CAD build for the part. Positions are in the model's coordinates, mm. A direction names the side the tool comes from. Round coordinates to 2 decimals unless told otherwise and drop trailing zeros. Order: outer loops, then holes, each group sorted by start corner. A loop starts at its lowest first (then second) coordinate and runs counter-clockwise, first axis right, second up. Notation, with made-up numbers: (-13.75, 85) - (27.25, 85) arc R25 ccw to (27.25, 114) - close; hole circle Ø3 at (85.25, 73.25). An arc over 180 degrees is marked (long way). Use one line per item in the form item = value. Start each with the question number.
from build123d import *

# Parameters (mm, degrees)
SKETCH_1_W               = 20
SKETCH_1_H               = 10
EXTRUDE_1_DEPTH          = 90
EXTRUDE_START            = -5
SKETCH_2_W               = 10
SKETCH_2_H               = 10
SKETCH_2_W_2             = 20
EXTRUDE_2_DEPTH          = 5
CUT_EXTRUDE_1_DEPTH      = 93.330926563
CUT_EXTRUDE_1_DEPTH_BACK = 93.330926563
SKETCH_3_R               = 2.75
FILLET_1_R               = 3


with BuildPart() as part:
    # 草图1 → 凸台-拉伸1 (new body)
    with BuildSketch(Plane.XY):
        with Locations((10, 5)):
            Rectangle(SKETCH_1_W, SKETCH_1_H)
    extrude(amount=EXTRUDE_1_DEPTH)

    # 草图2 → 凸台-拉伸2 (add)
    with BuildSketch(Plane(origin=(0, 0, 0), x_dir=(-1, 0, 0), z_dir=(0, 0, -1)).offset(EXTRUDE_START)):
        with Locations((-25, 5)):
            Rectangle(SKETCH_2_W, SKETCH_2_H)
        with Locations((-10, 15)):
            Rectangle(SKETCH_2_W_2, SKETCH_2_H)
        with Locations((5, 5)):
            Rectangle(SKETCH_2_W, SKETCH_2_H)
    extrude_2 = extrude(amount=-EXTRUDE_2_DEPTH)

    # 镜向1: 凸台-拉伸2 across plane
    add(extrude_2.mirror(Plane(origin=(0, 0, 45), x_dir=(1, 0, 0), z_dir=(0, 0, -1))))

    # 草图3 → 切除-拉伸1 (cut, two sides: drawn at the far end of the back side and taken through both)
    with BuildSketch(Plane(origin=(0, 0, 5), x_dir=(-1, 0, 0), z_dir=(0, 0, -1)).offset(-CUT_EXTRUDE_1_DEPTH_BACK)):
        with Locations(Location((5, 5, 0), (0, 0, 180))):
            Circle(SKETCH_3_R)
        with Locations(Location((-10, 15, 0), (0, 0, 180))):
            Circle(SKETCH_3_R)
        with Locations(Location((-25, 5, 0), (0, 0, 180))):
            Circle(SKETCH_3_R)
    extrude(amount=CUT_EXTRUDE_1_DEPTH + CUT_EXTRUDE_1_DEPTH_BACK, mode=Mode.SUBTRACT)

    # 圆角1
    # the kernel refuses this fillet: 3 mm, written as the material it takes off along each edge
    with BuildSketch(Plane(origin=(0, 10, -7.5), x_dir=(0, -1, 0), z_dir=(0, 0, 1)), Plane(origin=(0, 10, 85), x_dir=(0, -1, 0), z_dir=(0, 0, 1))) as fillet_1_piece_1:
        with BuildLine():
            CenterArc((FILLET_1_R, FILLET_1_R), FILLET_1_R, 180, 90)
            Line((0, FILLET_1_R), (0, 0))
            Line((0, 0), (FILLET_1_R, 0))
        make_face()
    extrude(amount=12.5, mode=Mode.SUBTRACT)
    with BuildSketch(Plane(origin=(20, 10, -7.5), x_dir=(0, -1, 0), z_dir=(0, 0, 1)), Plane(origin=(20, 10, 85), x_dir=(0, -1, 0), z_dir=(0, 0, 1))) as fillet_1_piece_2:
        with BuildLine():
            CenterArc((FILLET_1_R, -FILLET_1_R), FILLET_1_R, 90, 90)
            Line((0, -FILLET_1_R), (0, 0))
            Line((0, 0), (FILLET_1_R, 0))
        make_face()
    extrude(amount=12.5, mode=Mode.SUBTRACT)
    with BuildSketch(Plane(origin=(20, 20, -2.5), x_dir=(0, -1, 0), z_dir=(0, 0, 1)), Plane(origin=(30, 10, -2.5), x_dir=(0, -1, 0), z_dir=(0, 0, 1)), Plane(origin=(0, 20, 92.5), x_dir=(0, -1, 0), z_dir=(0, 0, -1)), Plane(origin=(-10, 10, 92.5), x_dir=(0, -1, 0), z_dir=(0, 0, -1))) as fillet_1_piece_3:
        with BuildLine():
            CenterArc((FILLET_1_R, -FILLET_1_R), FILLET_1_R, 90, 90)
            Line((0, -FILLET_1_R), (0, 0))
            Line((0, 0), (FILLET_1_R, 0))
        make_face()
    extrude(amount=20, mode=Mode.SUBTRACT)
    with BuildSketch(Plane(origin=(0, 20, -2.5), x_dir=(0, -1, 0), z_dir=(0, 0, 1)), Plane(origin=(-10, 10, -2.5), x_dir=(0, -1, 0), z_dir=(0, 0, 1)), Plane(origin=(30, 10, 92.5), x_dir=(0, -1, 0), z_dir=(0, 0, -1)), Plane(origin=(20, 20, 92.5), x_dir=(0, -1, 0), z_dir=(0, 0, -1))) as fillet_1_piece_4:
        with BuildLine():
            CenterArc((FILLET_1_R, FILLET_1_R), FILLET_1_R, 180, 90)
            Line((0, FILLET_1_R), (0, 0))
            Line((0, 0), (FILLET_1_R, 0))
        make_face()
    extrude(amount=20, mode=Mode.SUBTRACT)


solid = part.part
(1) Slice it at C-C (z = 6). Give the cut face in (x, y), and give its area (3 significant figures).
(2) Flat gauge pins, fed straight in: P1, Ø11, axis at x = 27, y = 3, coming from the +Z side; P2, Ø8, axis at y = 8.5, z = 15, coming from the +X side; P3, Ø3, axis at x = 9.5, y = 13.5, coming from the -Z side. Where does each tip first touch, or does it go through?
(3) Which spindle directions (+Z, -Z, +X, -X, +Y, -Y) get a long thin tool onto all of the face, cutting with end or side? Do faces 1 (the flat face through (10, 10, 87)), 2 (the flat face through (20, 13, 83)), 3 (the cylindrical face through (0.9, 9.14, 87.46)). Say none if no direction does.
(4) Slice it at B-B (x = 10). Give the cut face in (y, z).
(5) Slice it at A-A (y = 15). Give the cut face in (x, z).
(6) Mould opens along Z. For faces 4 (the cylindrical face through (-3.73, 7.44, 82.54)), 5 (the flat face through (10, 5, 0)), 6 (the flat face through (-2.7, 2.8, 10)) say: pulls with the +Z half, pulls with the -Z half, needs draft (parallel to the pull), parting line crosses it, or undercut.
(7) Slice it at D-D (x = -5). Give the cut face in (y, z).
(8) Wall check: line 1 (Y direction, x = 25, z = 82); line 2 (Z direction, x = -1, y = 3.5); line 3 (Y direction, x = 1.5, z = 41). Give the ranges that are in metal, low to high. Write a range as [from, to].
Results list:
q1.outline = (-10, 0) - (30, 0) - (30, 7) arc R3 ccw to (27, 10) - (20, 10) - (20, 17) arc R3 ccw to (17, 20) - (3, 20) arc R3 ccw to (0, 17) - (0, 10) - (-7, 10) arc R3 ccw to (-10, 7) - close; hole circle Ø5.5 at (-5, 5); hole circle Ø5.5 at (10, 15); hole circle Ø5.5 at (25, 5)
q1.area = 521 mm²
q2.P1 = 85
q2.P2 = 20
q2.P3 = 5
q3.face_1 = +Z, +X, -X, +Y
q3.face_2 = +Z, -Z, +X, +Y
q3.face_3 = +Z, -X, +Y
q4.outline = (0, 0) - (10, 0) - (10, 5) - (12.25, 5) - (12.25, 10) - (10, 10) - (10, 80) - (12.25, 80) - (12.25, 85) - (10, 85) - (10, 90) - (0, 90) - close; (17.75, 5) - (20, 5) - (20, 10) - (17.75, 10) - close; (17.75, 80) - (20, 80) - (20, 85) - (17.75, 85) - close
q5.outline = (0, 5) - (7.25, 5) - (7.25, 10) - (0, 10) - close; (0, 80) - (7.25, 80) - (7.25, 85) - (0, 85) - close; (12.75, 5) - (20, 5) - (20, 10) - (12.75, 10) - close; (12.75, 80) - (20, 80) - (20, 85) - (12.75, 85) - close
q6.face_4 = needs draft
q6.face_5 = pulls with the -Z half
q6.face_6 = undercut
q7.outline = (0, 5) - (2.25, 5) - (2.25, 10) - (0, 10) - close; (0, 80) - (2.25, 80) - (2.25, 85) - (0, 85) - close; (7.75, 5) - (10, 5) - (10, 10) - (7.75, 10) - close; (7.75, 80) - (10, 80) - (10, 85) - (7.75, 85) - close
q8.line_1 = [0, 2.25], [7.75, 10]
q8.line_2 = [5, 10], [80, 85]
q8.line_3 = [0, 10]
